Here's how the part is built. I have some questions about the finished solid (model axes, mm). Coordinates: 2 decimals unless noted, no trailing zeros. Write each loop counter-clockwise with the first axis right and the second up, starting at its lowest first coordinate (ties: lowest second). Pieces come first, ordered by that corner, then holes. Notation, with made-up numbers: M 43,-23 L 86,-23 A18 cw 86,5 Z; hole C 10.5,13.25 d6. An arc over 180 degrees is marked long. Use a Markdown table: item, result.
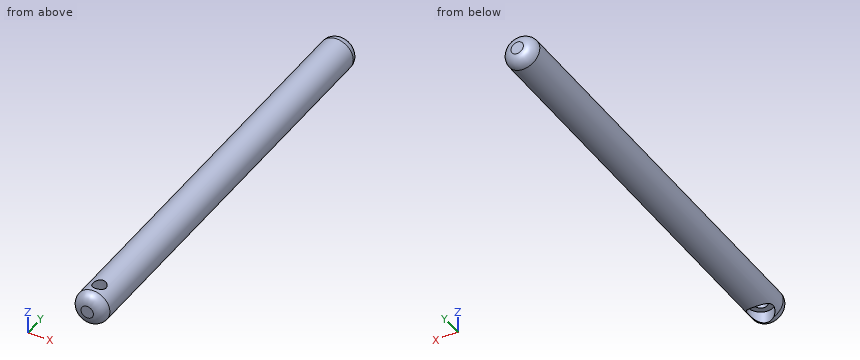
```python
from build123d import *

# Parameters (mm, degrees)
SKETCH1_R               = 4
BOSS_EXTRUDE1_DEPTH     = 105
CUT_EXTRUDE1_DEPTH      = 106.152270541
CUT_EXTRUDE1_DEPTH_BACK = 106.152270541
SKETCH2_R               = 1.6
CUT_EXTRUDE2_REACH      = 108.152
CUT_EXTRUDE2_END_RADIUS = 4
CUT_EXTRUDE2_START      = -1
SKETCH3_R               = 3
FILLET1_R               = 2.5


with BuildPart() as part:
    # Sketch1 → Boss-Extrude1 (new body)
    with BuildSketch(Plane(origin=(0, 0, 0), x_dir=(1, 0, 0), z_dir=(0, 1, 0))):
        with Locations(Location((0, 0, 0), (0, 0, 270))):
            Circle(SKETCH1_R)
    extrude(amount=BOSS_EXTRUDE1_DEPTH)

    # Sketch2 → Cut-Extrude1 (cut, two sides: drawn at the far end of the back side and taken through both)
    with BuildSketch(Plane.XY.offset(-CUT_EXTRUDE1_DEPTH_BACK)):
        with Locations(Location((0, 5, 0), (0, 0, 89.999999999))):
            Circle(SKETCH2_R)
    extrude(amount=CUT_EXTRUDE1_DEPTH + CUT_EXTRUDE1_DEPTH_BACK, mode=Mode.SUBTRACT)

    # Cut-Extrude2: up to this cylinder (the profile starts inside it)
    cut_extrude2_end = Plane(origin=(0, 5, 0), z_dir=(0, -1, 0)) * Cylinder(CUT_EXTRUDE2_END_RADIUS, 225.304, mode=Mode.PRIVATE)
    # Sketch3 → Cut-Extrude2 (cut, up to the surface)
    with BuildSketch(Plane.XY.offset(CUT_EXTRUDE2_START), mode=Mode.PRIVATE) as cut_extrude2_sk1:
        with Locations((0, 5)):
            Circle(SKETCH3_R)
    cut_extrude2_tool1 = extrude(cut_extrude2_sk1.sketch, amount=-CUT_EXTRUDE2_REACH, mode=Mode.PRIVATE) & cut_extrude2_end
    add(cut_extrude2_tool1.solids().sort_by_distance((0, 5, -1))[0], mode=Mode.SUBTRACT)

    # Fillet1
    # the kernel refuses this fillet: 2.5 mm, written as the material it takes off along each edge
    with BuildSketch(Plane(origin=(0, 0, 0), x_dir=(0, 0, 1), z_dir=(-1, 0, 0))) as fillet1_piece_1:
        with BuildLine():
            CenterArc((4 - FILLET1_R, FILLET1_R), FILLET1_R, 270, 90)
            Line((4 - FILLET1_R, 0), (4, 0))
            Line((4, 0), (4, FILLET1_R))
        make_face()
    revolve(axis=Axis((0, 0, 0), (0, 1, 0)), mode=Mode.SUBTRACT)
    with BuildSketch(Plane(origin=(0, 105, 0), x_dir=(0, 0, 1), z_dir=(-1, 0, 0))) as fillet1_piece_2:
        with BuildLine():
            CenterArc((4 - FILLET1_R, -FILLET1_R), FILLET1_R, 0, 90)
            Line((4 - FILLET1_R, 0), (4, 0))
            Line((4, 0), (4, -FILLET1_R))
        make_face()
    revolve(axis=Axis((0, 105, 0), (0, 1, 0)), mode=Mode.SUBTRACT)


solid = part.part
```
1. Will these pins go through, and if not, where does the flat tip stop? pin 1 Ø3 at (x, y) = (-2, 24) entering from +Z; pin 2 Ø3 at (x, y) = (-2, 67) entering from -Z.
Answers follow:
| item | result |
|---|---|
| pin 1 | stops at z = 3.97 |
| pin 2 | stops at z = -3.97 |
2. Suppose I cut it at B-B on y = 47. Write out the boundary of the cut face in (x, z), and give its area (3 significant figures).
Answers follow:
| item | result |
|---|---|
| outline | C 0,0 d8 |
| area | 50.3 mm2 |
3. I need wall thicknesses on probe 1 along X at (y, z) = (5, 1.25); probe 2 along X at (y, z) = (5, -1.75); probe 3 along Y at (x, z) = (0, -2.7). Which ranges of each line are inside material? Lowest first, please.
Answers follow:
| item | result |
|---|---|
| probe 1 | x = -3.8 to -1.6, 1.6 to 3.8 |
| probe 2 | x = -3.6 to -3, 3 to 3.6 |
| probe 3 | y = 0.31 to 2, 8 to 104.69 |
4. Suppose I cut it at A-A on y = 5. Write out the boundary of the cut face in (x, z), and give its area (3 significant figures).
Answers follow:
| item | result |
|---|---|
| outline | M -3,-2.65 L -3,-1 L -1.6,-1 L -1.6,3.67 A4 ccw Z; M 1.6,-1 L 3,-1 L 3,-2.65 A4 ccw 1.6,3.67 Z |
| area | 19.1 mm2 |
